Study the drawing (mm; zero at the part's minimum x, y, z) and answer. Coordinates: 2 decimals unless noted, no trailing zeros. Order: outer loops, then holes, each group sorted by start corner. A loop starts at its lowest first (then second) coordinate and runs counter-clockwise, first axis right, second up. Notation, with made-up numbers: M -15,49 L 13,49 A30 ccw 13,83 Z; hole C 58,58 d9. An arc over 180 degrees is marked long. One line per item, written item: value. Start each with the question number.
Q1. The part is cut by section C-C on y = 9.75. Give the vertices of the cut face in (x, z).
Q2. Straight lines are drawn through the part: line 1 along Z through (x, y) = (7, 13.5); line 2 along X through (y, z) = (6.5, 18); line 3 along X through (y, z) = (8.25, 15) (1 decimal). For each, find the intervals that lie inside material, in ascending order. Write a range as [from, to].
Q3. The part is cut by section A-A on z = 2.25. Give the number of separate pieces and of enclosed holes in the cut face, then the cut area to 3 significant figures.
Q4. Each of these flat-tipped pins is pushed along its axis until it touches: pin 1 Ø10 at (x, z) = (23.5, 16.5) entering from -Y; pin 2 Ø3 at (x, y) = (4.5, 7.5) entering from +Z; pin 3 Ø10 at (x, z) = (10.5, 19) entering from +Y. Where does it stop, or does it pass through?
Q5. The part is cut by section D-D on y = 2.75. Give the vertices of the cut face in (x, z), then the cut area to 3 significant figures.
Q6. Determine the mould class of the marked faces 1, 2 and 3 for opening direction X: pulls with the +X half, pulls with the -X half, needs draft (parallel to the pull), parting line crosses it, or undercut.
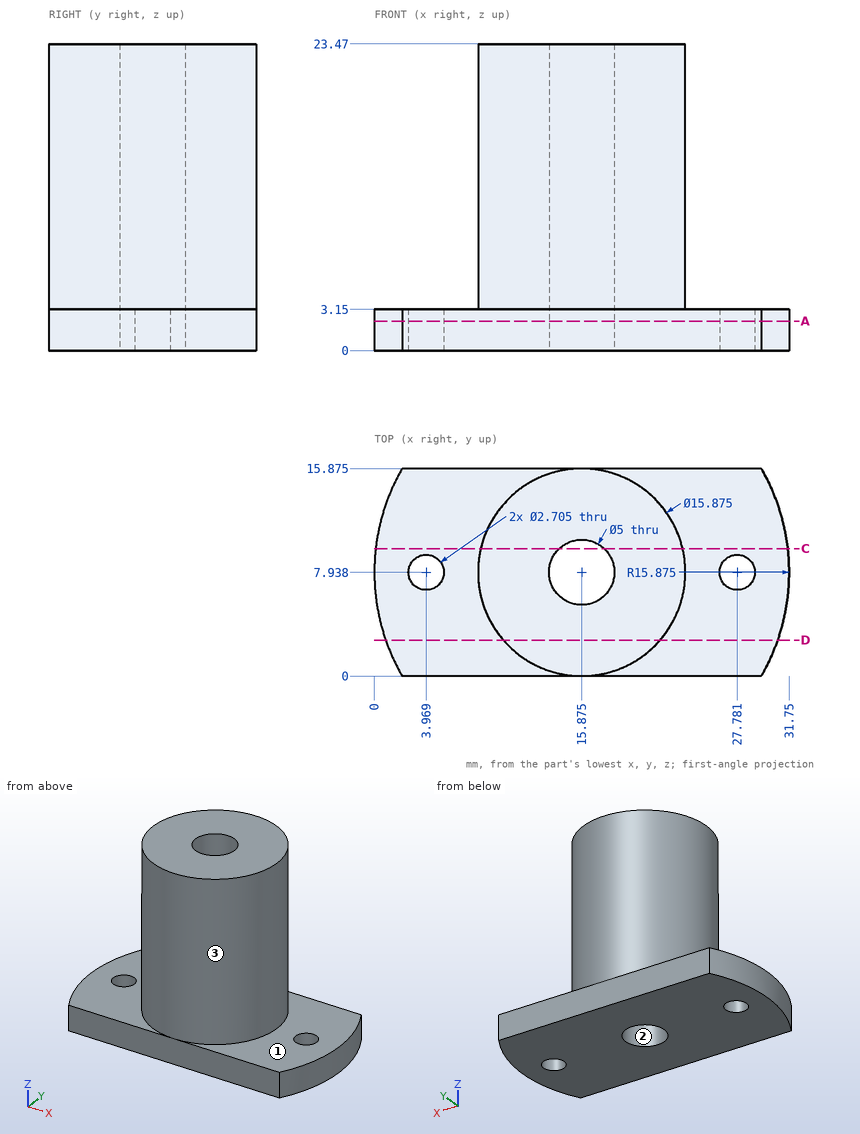
Output:
1. outline: M 0.1,0 L 14.15,0 L 14.15,23.47 L 8.15,23.47 L 8.15,3.15 L 0.1,3.15 Z; M 17.6,0 L 31.65,0 L 31.65,3.15 L 23.6,3.15 L 23.6,23.47 L 17.6,23.47 Z
2. line 1: z = [0, 3.15]
2. line 2: x = [8.07, 13.83], [17.92, 23.68]
2. line 3: x = [7.9, 13.4], [18.4, 23.8]
3. separate pieces: 1
3. enclosed holes: 3
3. area: 451 mm^2
4. pin 1: stops at y = 0.45
4. pin 2: stops at z = 3.15
4. pin 3: stops at y = 15.87
5. outline: M 0.87,0 L 30.88,0 L 30.88,3.15 L 21.88,3.15 L 21.88,23.47 L 9.87,23.47 L 9.87,3.15 L 0.87,3.15 Z
5. area: 339 mm^2
6. face 1: needs draft
6. face 2: undercut
6. face 3: parting line crosses it
